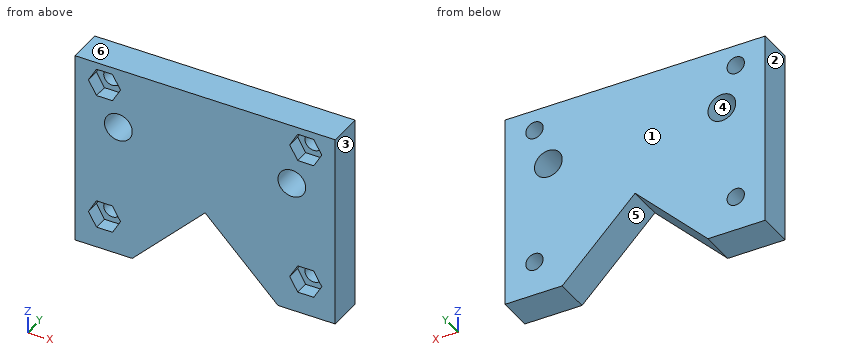
from build123d import *

# Parameters (mm, degrees)
SKETCH1_W               = 75
SKETCH1_H               = 10
BOSS_EXTRUDE1_DEPTH     = 35
CUT_EXTRUDE1_DEPTH      = 53.261362401
CUT_EXTRUDE1_DEPTH_BACK = 53.261362401
SKETCH2_R               = 4
CUT_EXTRUDE2_DEPTH      = 53.261362401
CUT_EXTRUDE2_DEPTH_BACK = 53.261362401
SKETCH3_R               = 2.5
SKETCH4_W               = 75
SKETCH4_H               = 10
BOSS_EXTRUDE2_DEPTH     = 21
CUT_EXTRUDE3_DEPTH      = 53.261362401
CUT_EXTRUDE3_DEPTH_BACK = 53.261362401
SKETCH5_R               = 2.5
CUT_EXTRUDE4_DEPTH      = 4
CUT_EXTRUDE5_DEPTH      = 53.261362401
CUT_EXTRUDE5_DEPTH_BACK = 53.261362401


with BuildPart() as part:
    # Sketch1 → Boss-Extrude1 (new body)
    with BuildSketch(Plane.XY):
        with Locations((0, -5)):
            Rectangle(SKETCH1_W, SKETCH1_H)
    extrude(amount=BOSS_EXTRUDE1_DEPTH)

    # Sketch2 → Cut-Extrude1 (cut, two sides: drawn at the far end of the back side and taken through both)
    with BuildSketch(Plane(origin=(0, 0, 0), x_dir=(1, 0, 0), z_dir=(0, 1, 0)).offset(-CUT_EXTRUDE1_DEPTH_BACK)):
        with Locations(Location((-25, -17.5, 0), (0, 0, 180))):
            Circle(SKETCH2_R)
        with Locations(Location((25, -17.5, 0), (0, 0, 180))):
            Circle(SKETCH2_R)
    extrude(amount=CUT_EXTRUDE1_DEPTH + CUT_EXTRUDE1_DEPTH_BACK, mode=Mode.SUBTRACT)

    # Sketch3 → Cut-Extrude2 (cut, two sides: drawn at the far end of the back side and taken through both)
    with BuildSketch(Plane(origin=(0, 0, 0), x_dir=(1, 0, 0), z_dir=(0, 1, 0)).offset(-CUT_EXTRUDE2_DEPTH_BACK)):
        with Locations(Location((-29, -29, 0), (0, 0, 180))):
            Circle(SKETCH3_R)
        with Locations((29, -29)):
            Circle(SKETCH3_R)
    extrude(amount=CUT_EXTRUDE2_DEPTH + CUT_EXTRUDE2_DEPTH_BACK, mode=Mode.SUBTRACT)

    # Sketch4 → Boss-Extrude2 (add)
    with BuildSketch(Plane(origin=(0, 0, 0), x_dir=(-1, 0, 0), z_dir=(0, 0, -1))):
        with Locations((0, -5)):
            Rectangle(SKETCH4_W, SKETCH4_H)
    extrude(amount=BOSS_EXTRUDE2_DEPTH)

    # Sketch5 → Cut-Extrude3 (cut, two sides: drawn at the far end of the back side and taken through both)
    with BuildSketch(Plane(origin=(0, 0, 0), x_dir=(1, 0, 0), z_dir=(0, 1, 0)).offset(-CUT_EXTRUDE3_DEPTH_BACK)):
        with Locations(Location((-29, 11, 0), (0, 0, 180))):
            Circle(SKETCH5_R)
        with Locations((29, 11)):
            Circle(SKETCH5_R)
    extrude(amount=CUT_EXTRUDE3_DEPTH + CUT_EXTRUDE3_DEPTH_BACK, mode=Mode.SUBTRACT)

    # Sketch6 → Cut-Extrude4 (cut)
    with BuildSketch(Plane.XZ.offset(10)):
        Polygon((-24.381197846, 29), (-26.690598923, 33), (-31.309401077, 33), (-33.618802154, 29), (-31.309401077, 25), (-26.690598923, 25), align=None)
        Polygon((33.618802154, 29), (31.309401077, 33), (26.690598923, 33), (24.381197846, 29), (26.690598923, 25), (31.309401077, 25), align=None)
        Polygon((-24.381197846, -11), (-26.690598923, -7), (-31.309401077, -7), (-33.618802154, -11), (-31.309401077, -15), (-26.690598923, -15), align=None)
        Polygon((33.618802154, -11), (31.309401077, -7), (26.690598923, -7), (24.381197846, -11), (26.690598923, -15), (31.309401077, -15), align=None)
    extrude(amount=-CUT_EXTRUDE4_DEPTH, mode=Mode.SUBTRACT)

    # Sketch7 → Cut-Extrude5 (cut, two sides: drawn at the far end of the back side and taken through both)
    with BuildSketch(Plane(origin=(0, 0, 0), x_dir=(1, 0, 0), z_dir=(0, 1, 0)).offset(-CUT_EXTRUDE5_DEPTH_BACK)):
        Polygon((0, 0), (21, 21), (-21, 21), align=None)
    extrude(amount=CUT_EXTRUDE5_DEPTH + CUT_EXTRUDE5_DEPTH_BACK, mode=Mode.SUBTRACT)


solid = part.part
Check sheet for the modelled part. Datum: model origin and axes. Units: mm. Face numbers are marked on the shaded views. A direction names the side the tool comes from. Round coordinates to 2 decimals unless told otherwise and drop trailing zeros. Order: outer loops, then holes, each group sorted by start corner. A loop starts at its lowest first (then second) coordinate and runs counter-clockwise, first axis right, second up.
(1) Go/stop test with flat-tipped pins: P1, Ø2.5, axis at x = 30.5, z = 28.5, coming from the -Y side; P2, Ø1, axis at x = -19.5, y = -7.5, coming from the -Z side. Record where each tip stops, or that it passes through.
(2) Access from +Z, -Z, +X, -X, +Y, -Y to the whole of each face (thin tool, end or side, straight path). Record for the marked faces 5 and 6.
(3) Cross-section at D-D, the plane z = -10. Enter the section's corners in (x, y).
(4) Cross-section at A-A, the plane z = 17.5. Enter the section's corners in (x, y).
(5) Draft check along X on the marked faces 1, 2, 3 and 4. Enter one of: pulls with the +X half, pulls with the -X half, needs draft (parallel to the pull), parting line crosses it, or undercut.
(6) Scan lines: probe 1 along X at (y, z) = (-3.75, 30); probe 2 along X at (y, z) = (-3.5, 17.5); probe 3 along X at (y, z) = (-9, -12.5). Record each from-to range of solid material in increasing order.
(7) Cross-section at B-B, the plane x = 22.5. Enter the section's corners in (y, z), and give its area (3 significant figures).
(8) Cross-section at C-C, the plane y = -2.5. Enter the section's corners in (x, z), and give its area (3 significant figures).
Check sheet entries:
1. P1: stops at y = -6
1. P2: stops at z = -20
2. face 5: -Z, +Y, -Y
2. face 6: +Z, +X, -X, +Y, -Y
3. outline: (-37.5, -10) - (-33.04, -10) - (-33.04, -6) - (-31.29, -6) - (-31.29, 0) - (-37.5, 0) - close; (-26.71, -6) - (-24.96, -6) - (-24.96, -10) - (-10, -10) - (-10, 0) - (-26.71, 0) - close; (10, -10) - (24.96, -10) - (24.96, -6) - (26.71, -6) - (26.71, 0) - (10, 0) - close; (31.29, -6) - (33.04, -6) - (33.04, -10) - (37.5, -10) - (37.5, 0) - (31.29, 0) - close
4. outline: (-37.5, -10) - (-29, -10) - (-29, 0) - (-37.5, 0) - close; (-21, -10) - (21, -10) - (21, 0) - (-21, 0) - close; (29, -10) - (37.5, -10) - (37.5, 0) - (29, 0) - close
5. face 1: needs draft
5. face 2: pulls with the -X half
5. face 3: pulls with the +X half
5. face 4: undercut
6. probe 1: x = -37.5 to -31.29, -26.71 to 26.71, 31.29 to 37.5
6. probe 2: x = -37.5 to -29, -21 to 21, 29 to 37.5
6. probe 3: x = -37.5 to -32.75, -25.25 to -12.5, 12.5 to 25.25, 32.75 to 37.5
7. outline: (-10, -21) - (0, -21) - (0, 14.38) - (-10, 14.38) - close; (-10, 20.62) - (0, 20.62) - (0, 35) - (-10, 35) - close
7. area: 498 mm2
8. outline: (-37.5, -21) - (-21, -21) - (0, 0) - (21, -21) - (37.5, -21) - (37.5, 35) - (-37.5, 35) - close; hole circle Ø5 at (-29, -11); hole circle Ø5 at (-29, 29); hole circle Ø8 at (-25, 17.5); hole circle Ø8 at (25, 17.5); hole circle Ø5 at (29, -11); hole circle Ø5 at (29, 29)
8. area: 3,580 mm2
